```python
from build123d import *

# Parameters (mm, degrees)
ESQUISSE1_R        = 6.35
ESQUISSE1_R_2      = 9.5
BOSS_EXTRU_1_DEPTH = 28.5


with BuildPart() as part:
    # Esquisse1 → Boss.-Extru.1 (new body)
    with BuildSketch(Plane.XY):
        with BuildLine():
            Line((-74.269831122, -14.050908363), (-69.549469101, -62.162426551))
            ThreePointArc((-69.549469101, -62.162426551), (-62.431950288, -76.312412018), (-47.654598332, -82.014256626))
            Line((-47.654598332, -82.014256626), (11.345401668, -82.014256626))
            Line((11.345401668, -82.014256626), (11.345401668, -63.751175412))
            Line((11.345401668, -63.751175412), (-10.654598332, -63.751175412))
            ThreePointArc((-10.654598332, -63.751175412), (-14.391517119, -60.014256626), (-10.654598332, -56.27733784))
            Line((-10.654598332, -56.27733784), (11.345401668, -56.27733784))
            Line((11.345401668, -56.27733784), (11.345401668, -46.014256626))
            ThreePointArc((11.345401668, -46.014256626), (-23.716977968, -34.858356839), (-47.601181026, -6.869619639))
            ThreePointArc((-47.601181026, -6.869619639), (-63.976959265, 0.834568173), (-74.269831122, -14.050908363))
        make_face()
        with Locations(Location((-60.336723839, -12.683889074, 0), (0, 0, 180))):
            Circle(ESQUISSE1_R, mode=Mode.SUBTRACT)
        with Locations(Location((-47.654598332, -60.014256626, 0), (0, 0, 180))):
            Circle(ESQUISSE1_R_2, mode=Mode.SUBTRACT)
    extrude(amount=BOSS_EXTRU_1_DEPTH)


solid = part.part
```
Can you work these out from the model? Positions are in its coordinate system, mm. A direction names the side the tool comes from. Round coordinates to 2 decimals unless told otherwise and drop trailing zeros. Loops run counter-clockwise (first coordinate to the right, second up) from the corner with the lowest first, then second, coordinate; pieces in that order, holes last. Notation, with made-up numbers: (21, 37) -> (40, 37) arc R16 cw to (40, 52) -> close; hole circle Ø5 at (54.25, 36). An arc over 180 degrees is marked (long way). One line per item, written item: value. Start each with the question number.
1. If we section it at B-B, the plane x = 5: Write out the boundary of the cut face in (y, z), then the cut area to 3 significant figures.
2. If we mould it in two halves opening along Y, with no side actions, what happens to faces 3 (the cylindrical face through (-14.39, -60.1, 14.05)), 4 (the flat face through (11.345, -73, 14)), 5 (the flat face through (-71.943, -37.77, 14.05))? For each: pulls with the +Y half, pulls with the -Y half, needs draft (parallel to the pull), parting line crosses it, or undercut.
3. If I drill on probe 1 along Y at (x, z) = (-56, 15.25); probe 2 along X at (y, z) = (-65.5, 3.75); probe 3 along Y at (x, z) = (-43.5, 18.5), over which ranges is the centre line in solid material (lowest first)?
4. If we section it at C-C, the plane z = 7: Write out the boundary of the cut face in (x, y).
5. If we section it at A-A, the plane y = -10.5: Write out the boundary of the cut face in (x, z).
6. For faces 1 (the cylindrical face through (-23.281, -35.145, 14.05)), 2 (the flat face through (0, -63.751, 14)), which set-ups out of +Z, -Z, +X, -X, +Y, -Y let a thin tool reach every point of the face, with its end or its side?
7. If we section it at D-D, the plane y = -40: Write out the boundary of the cut face in (x, z).
8. For pin 1 (6 mm diameter, centred on y = -49.5, z = 21.5, fed in from -X); pin 2 (4 mm diameter, centred on x = -24.5, z = 12, fed in from +Y); pin 3 (5 mm diameter, centred on x = -58.5, z = 11, fed in from -Y), each with a flat end and sliding along its axis, tell me the tip position at first contact or that it passes through.
Calculated:
1. outline: (-82.01, 0) -> (-63.75, 0) -> (-63.75, 28.5) -> (-82.01, 28.5) -> close; (-56.28, 0) -> (-45.52, 0) -> (-45.52, 28.5) -> (-56.28, 28.5) -> close
1. area: 827 mm²
2. face 3: undercut
2. face 4: needs draft
2. face 5: pulls with the -Y half
3. probe 1: y = -80.37 to -64.55, -55.48 to -17.32, -8.05 to 0.63
3. probe 2: x = -68.96 to -55.41, -39.9 to 11.35
3. probe 3: y = -82.01 to -68.56, -51.47 to -14.5
4. outline: (-74.27, -14.05) -> (-69.55, -62.16) arc R22 ccw to (-47.65, -82.01) -> (11.35, -82.01) -> (11.35, -63.75) -> (-10.65, -63.75) arc R3.74 cw to (-10.65, -56.28) -> (11.35, -56.28) -> (11.35, -46.01) arc R67 cw to (-47.6, -6.87) arc R14 ccw to start; hole circle Ø12.7 at (-60.34, -12.68); hole circle Ø19 at (-47.65, -60.01)
5. outline: (-74.17, 0) -> (-66.3, 0) -> (-66.3, 28.5) -> (-74.17, 28.5) -> close; (-54.37, 0) -> (-45.81, 0) -> (-45.81, 28.5) -> (-54.37, 28.5) -> close
6. face 1: +Z, -Z, +X, +Y
6. face 2: +Z, -Z, +X
7. outline: (-71.72, 0) -> (-14.46, 0) -> (-14.46, 28.5) -> (-71.72, 28.5) -> close
8. pin 1: stops at x = -71.09
8. pin 2: stops at y = -32.91
8. pin 3: stops at y = -80.37
